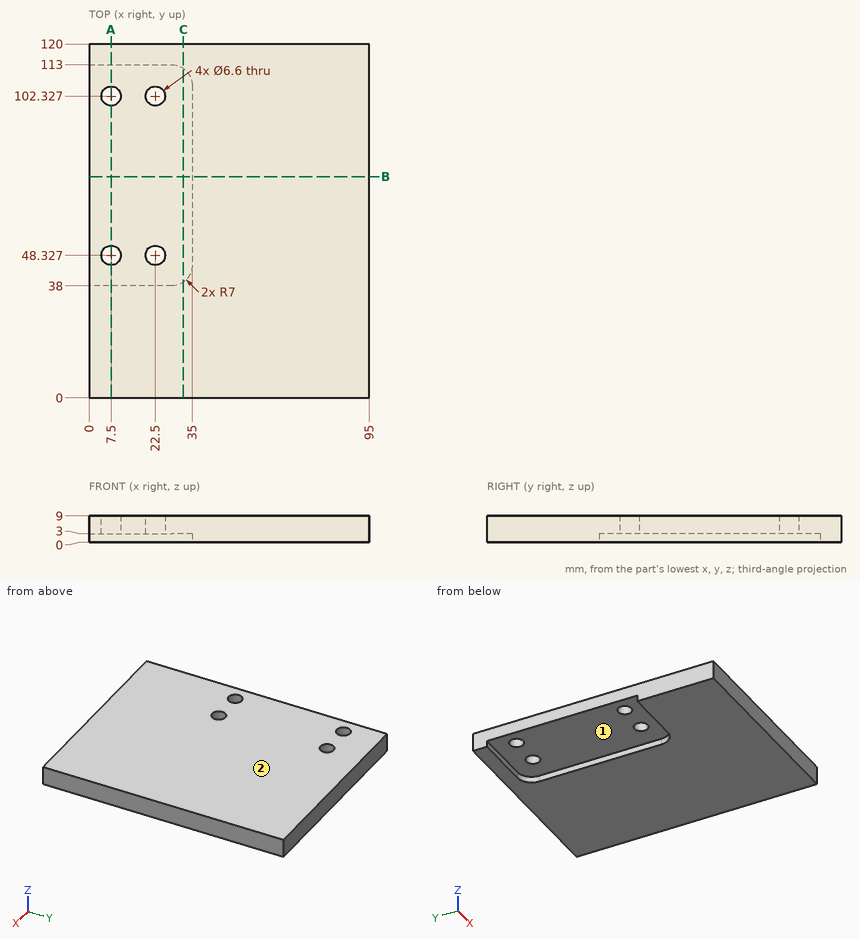
Job drawing, mm, ordinate dimensions from the low corner. One solid piece. Round coordinates to 2 decimals unless told otherwise and drop trailing zeros. Loops run counter-clockwise (first coordinate to the right, second up) from the corner with the lowest first, then second, coordinate; pieces in that order, holes last.
(1) Cut at A-A (x = 7.5). Give the cut face in (y, z), plus the area to 3 significant figures.
(2) Two-plate mould, pull along Y, no slides. Class the marked faces 1 and 2: +Y half, -Y half, draft (parallel to the pull), parting line (faces both ways), or undercut.
(3) Cut at C-C (x = 32). Give the cut face in (y, z).
(4) Wall check: line 1 along Y through (x, z) = (22.5, 6.95); line 2 along Y through (x, z) = (8.5, 4); line 3 along X through (y, z) = (47, 6.25). Give the ranges that are in metal, low to high.
(5) Drop flat-ended pins along their axis: pin 1 (4 mm diameter, centred on x = 22.5, y = 48.33, fed in from -Z); pin 2 (10.5 mm diameter, centred on x = 7.5, y = 102.33, fed in from -Z); pin 3 (2.5 mm diameter, centred on y = 87.5, z = 1.5, fed in from -X). Give the stop position or say it passes through.
(6) Cut at B-B (y = 75). Give the cut face in (x, z).
Findings below:
1. outline: (0, 0) - (38, 0) - (38, 3) - (45.03, 3) - (45.03, 9) - (0, 9) - close; (51.63, 3) - (99.03, 3) - (99.03, 9) - (51.63, 9) - close; (105.63, 3) - (113, 3) - (113, 0) - (120, 0) - (120, 9) - (105.63, 9) - close
1. area: 776 mm2
2. face 1: undercut
2. face 2: draft
3. outline: (0, 0) - (39.26, 0) - (39.26, 3) - (111.74, 3) - (111.74, 0) - (120, 0) - (120, 9) - (0, 9) - close
4. line 1: y = 0 to 45.03, 51.63 to 99.03, 105.63 to 120
4. line 2: y = 0 to 45.18, 51.47 to 99.18, 105.47 to 120
4. line 3: x = 0 to 4.48, 10.52 to 19.48, 25.52 to 95
5. pin 1: passes through
5. pin 2: stops at z = 3
5. pin 3: stops at x = 35
6. outline: (0, 3) - (35, 3) - (35, 0) - (95, 0) - (95, 9) - (0, 9) - close
